```python
from build123d import *

# Parameters (mm, degrees)
SKETCH_1_W           = 2.54
SKETCH_1_H           = 6.2
EXTRUDE_1_DEPTH      = 3
SKETCH_2_W           = 1.2
SKETCH_2_H           = 2
CUT_EXTRUDE_1_DEPTH  = 0.5
SKETCH_3_W           = 1
SKETCH_3_H           = 1
EXTRUDE_1_2_DEPTH    = 1
FILLET_1_R           = 0.3
CHAMFER_1_SIZE       = 0.4
CHAMFER_1_SIZE2      = 1.098990968
EXTRUDE_2_DEPTH      = 0.45
EXTRUDE_2_DEPTH_BACK = 0.45
SKETCH_5_W           = 0.25
SKETCH_5_H           = 1.121567526
CUT_EXTRUDE_2_DEPTH  = 9.661137339


with BuildPart() as part:
    # 草图1 → Extrude 1 (new body)
    with BuildSketch(Plane(origin=(0, 0, 0), x_dir=(1, 0, 0), z_dir=(0, 1, 0))):
        Rectangle(SKETCH_1_W, SKETCH_1_H)
    extrude(amount=EXTRUDE_1_DEPTH)

    # 草图2 → 切除-拉伸1 (cut)
    with BuildSketch(Plane(origin=(0, 3, 0), x_dir=(1, 0, 0), z_dir=(0, 1, 0))):
        Rectangle(SKETCH_2_W, SKETCH_2_H)
    extrude(amount=-CUT_EXTRUDE_1_DEPTH, mode=Mode.SUBTRACT)

    # 草图3 → Extrude 1 2 (add)
    with BuildSketch(Plane(origin=(0, 2.5, 0), x_dir=(1, 0, 0), z_dir=(0, 1, 0))):
        with Locations((0, 0.4)):
            Rectangle(SKETCH_3_W, SKETCH_3_H)
    extrude(amount=EXTRUDE_1_2_DEPTH)

    # 圆角1
    fillet_1_edges = [part.edges().sort_by_distance(p)[0] for p in [
        (0, 3, -3.1),
        (0, 3, 3.1),
    ]]
    fillet(fillet_1_edges, radius=FILLET_1_R)

    # 倒角1
    chamfer_1_edges = [part.edges().sort_by_distance(p)[0] for p in [
        (0, 0, -3.1),
        (0, 0, 3.1),
    ]]
    chamfer_1_side = [part.faces().sort_by_distance(p)[0] for p in [
        (0, 0, 0),
    ]]
    chamfer(chamfer_1_edges, length=CHAMFER_1_SIZE, length2=CHAMFER_1_SIZE2, reference=chamfer_1_side[0])

    # 草图4 → 凸台-拉伸2 (add, two sides: drawn at the far end of the back side and taken through both)
    with BuildSketch(Plane(origin=(0, 0, 0), x_dir=(0, 0, -1), z_dir=(1, 0, 0)).offset(-EXTRUDE_2_DEPTH_BACK)):
        Polygon((-2.805439179, 1.628598981), (-3.91, 1.628598981), (-3.91, -1.548691293), (-3.71, -1.548691293), (-3.71, 1.428598981), (-2.805439179, 1.428598981), align=None)
        Polygon((2.805439179, 1.428598981), (2.805439179, 1.628598981), (3.91, 1.628598981), (3.91, -1.548691293), (3.71, -1.548691293), (3.71, 1.428598981), align=None)
    extrude(amount=EXTRUDE_2_DEPTH + EXTRUDE_2_DEPTH_BACK)

    # 草图5 → 切除-拉伸2 (cut, through all)
    with BuildSketch(Plane.XY.offset(3.91)):
        with Locations((0.325, -0.98790753)):
            Rectangle(SKETCH_5_W, SKETCH_5_H)
        with Locations((-0.325, -0.98790753)):
            Rectangle(SKETCH_5_W, SKETCH_5_H)
    extrude(amount=-CUT_EXTRUDE_2_DEPTH, mode=Mode.SUBTRACT)


solid = part.part
```
Read the model definition and answer for the solid it produces. Units are mm, in the model's axes. A direction names the side the tool comes from. Coordinates: 2 decimals unless noted, no trailing zeros. Order: outer loops, then holes, each group sorted by start corner. A loop starts at its lowest first (then second) coordinate and runs counter-clockwise, first axis right, second up. Notation, with made-up numbers: (71, 66.25) - (114, 66.25) arc R30 ccw to (114, 105.25) - close; hole circle Ø5 at (13, 26). An arc over 180 degrees is marked (long way). Answer as a JSON object with one key per item and string values. Group by question number.
Item 1: Section A-A (y = -1.1) is taken. Give the vertices of the cut face in (x, z).
Item 2: Section D-D (z = 2) is taken. Give the vertices of the cut face in (x, y), plus the area to 3 significant figures.
Item 3: Section C-C (y = 0.9) is taken. Give the vertices of the cut face in (x, z).
Item 4: The mould has two halves that part along X. Classify faces 1 (the face through (0, 3, 0.1)), 2 (the face through (1.27, 1, 0)), 3 (the face through (-0.018, 0.557, 2.903)): +X half, -X half, draft (parallel to the pull), parting line (faces both ways), or undercut.
Item 5: Consider probe 1 along Z at (x, y) = (0.25, 0.8); probe 2 along Z at (x, y) = (-0.55, 2.2); probe 3 along Z at (x, y) = (0.4, 0.25). Determine where each line is inside the solid, lowest interval first. Write a range as from..to.
Item 6: A tool of negligible diameter and unlimited length cuts with its end or side. For faces 4 (the face through (-1.27, 1, 0)), 5 (the face through (0, 3.5, -0.4)), 6 (the face through (0, 1.629, -3.5)), 7 (the face through (-0.018, 0.557, -2.903)), 8 (the face through (0, 1.629, 3.5)), from which of +Z, -Z, +X, -X, +Y, -Y can it reach the whole face along a straight path? Write none if from no direction.
Item 7: Section B-B (x = -1.1) is taken. Give the vertices of the cut face in (y, z), plus the area to 3 significant figures.
Item 8: Flat-ended cylindrical pins translate along their axes: P1, Ø0.9, axis at y = 0.5, z = -3.5, coming from the -X side; P2, Ø1.5, axis at x = 0.5, z = -2, coming from the -Y side; P3, Ø0.6, axis at x = 0.5, y = 2.5, coming from the +Z side. Find the tip coordinate at first contact, or state that the pin passes through.
Results are:
{
 "1": {"outline": "(-0.2, -3.91) - (0.2, -3.91) - (0.2, -3.71) - (-0.2, -3.71) - close; (-0.2, 3.71) - (0.2, 3.71) - (0.2, 3.91) - (-0.2, 3.91) - close"},
 "2": {"outline": "(-1.27, 0) - (1.27, 0) - (1.27, 3) - (-1.27, 3) - close", "area": "7.62 mm^2"},
 "3": {"outline": "(-1.27, -3.03) - (1.27, -3.03) - (1.27, 3.03) - (-1.27, 3.03) - close; (-0.45, -3.91) - (0.45, -3.91) - (0.45, -3.71) - (-0.45, -3.71) - close; (-0.45, 3.71) - (0.45, 3.71) - (0.45, 3.91) - (-0.45, 3.91) - close"},
 "4": {"face 1": "undercut", "face 2": "+X half", "face 3": "draft"},
 "5": {"probe 1": "z = -3.91..-3.71, -2.99..2.99, 3.71..3.91", "probe 2": "z = -3.1..3.1", "probe 3": "z = -3.91..-3.71, -2.79..2.79, 3.71..3.91"},
 "6": {"face 4": "+Z, -Z, -X, +Y, -Y", "face 5": "+Z, -Z, +X, -X, +Y", "face 6": "-Z, +X, -X, +Y", "face 7": "+X, -X, -Y", "face 8": "+Z, +X, -X, +Y"},
 "7": {"outline": "(0, -2.7) - (1.1, -3.1) - (2.7, -3.1) arc R0.3 ccw to (3, -2.8) - (3, 2.8) arc R0.3 ccw to (2.7, 3.1) - (1.1, 3.1) - (0, 2.7) - close", "area": "18.1 mm^2"},
 "8": {"P1": "stops at x = -0.45", "P2": "stops at y = 0", "P3": "stops at z = 3.1"}
}
